Input: dimensioned drawing with shaded views. Units: mm. Origin: part minimum x, y, z. A direction names the side the tool comes from. Round coordinates to 2 decimals unless told otherwise and drop trailing zeros. Loops run counter-clockwise (first coordinate to the right, second up) from the corner with the lowest first, then second, coordinate; pieces in that order, holes last. Notation, with made-up numbers: (82, 62.25) -> (115, 62.25) arc R21 cw to (115, 99.25) -> close; hole circle Ø7 at (16.25, 40.25). An arc over 180 degrees is marked (long way). Answer as a JSON object with one key per item and string values.
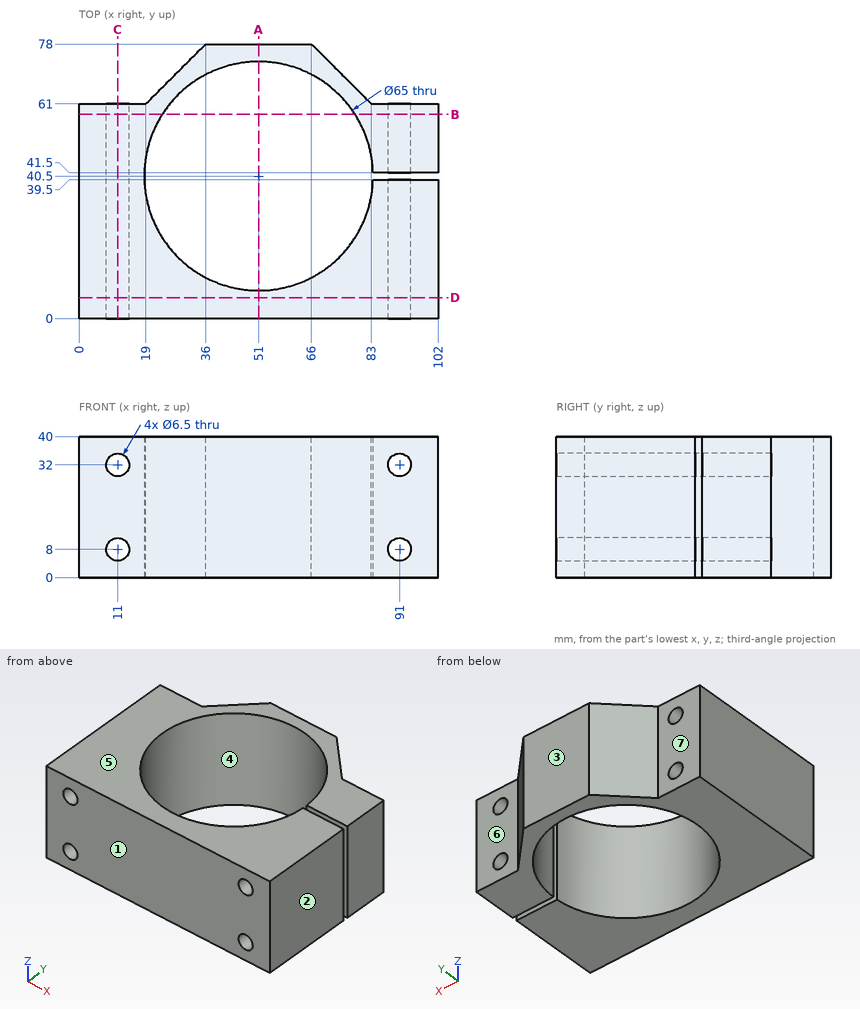
1) Reachability of the marked faces 5, 6 and 7 from +Z, -Z, +X, -X, +Y, -Y: full face, straight path, thin tool, end or side. Return the list, or none.
Output:
{"face 5": "+Z, +X, -X, +Y, -Y", "face 6": "+Z, -Z, +X, +Y", "face 7": "+Z, -Z, -X, +Y"}
2) Section B-B, the plane y = 58. Output: boundary loops of the cut face in (x, z).
Output:
{"outline": "(0, 0) -> (23.61, 0) -> (23.61, 40) -> (0, 40) -> close; (78.39, 0) -> (102, 0) -> (102, 40) -> (78.39, 40) -> close; hole circle Ø6.5 at (11, 8); hole circle Ø6.5 at (11, 32); hole circle Ø6.5 at (91, 8); hole circle Ø6.5 at (91, 32)"}
3) Draft query along Y for the marked faces 1, 2, 3 and 4. Return one class per face: +Y half, -Y half, draft (parallel to the pull), parting line (faces both ways), or undercut.
Output:
{"face 1": "-Y half", "face 2": "draft", "face 3": "+Y half", "face 4": "undercut"}
4) Ray query, probe 1 along X at (y, z) = (14, 32); probe 2 along Z at (x, y) = (8.5, 8); probe 3 along Y at (x, z) = (51, 15). Return the intervals inside material, ascending.
Output:
{"probe 1": "x = 0 to 7.75, 14.25 to 32.19, 69.81 to 87.75, 94.25 to 102", "probe 2": "z = 0 to 5.92, 10.08 to 29.92, 34.08 to 40", "probe 3": "y = 0 to 8, 73 to 78"}
5) Section C-C, the plane x = 11. Output: boundary loops of the cut face in (y, z), plus the area to 3 significant figures.
Output:
{"outline": "(0, 0) -> (61, 0) -> (61, 4.75) -> (0, 4.75) -> close; (0, 11.25) -> (61, 11.25) -> (61, 28.75) -> (0, 28.75) -> close; (0, 35.25) -> (61, 35.25) -> (61, 40) -> (0, 40) -> close", "area": "1,650 mm^2"}
6) Contact query for a flat-ended pin moving along its axis: P1, Ø15, axis at x = 7.5, z = 26.5, coming from the +Y side. Output: stop coordinate, or through.
Output:
{"P1": "stops at y = 61"}
7) Section A-A, the plane x = 51. Output: boundary loops of the cut face in (y, z), plus the area to 3 significant figures.
Output:
{"outline": "(0, 0) -> (8, 0) -> (8, 40) -> (0, 40) -> close; (73, 0) -> (78, 0) -> (78, 40) -> (73, 40) -> close", "area": "520 mm^2"}
8) Section D-D, the plane y = 6. Output: boundary loops of the cut face in (x, z), plus the area to 3 significant figures.
Output:
{"outline": "(0, 0) -> (102, 0) -> (102, 40) -> (0, 40) -> close; hole circle Ø6.5 at (11, 8); hole circle Ø6.5 at (11, 32); hole circle Ø6.5 at (91, 8); hole circle Ø6.5 at (91, 32)", "area": "3,950 mm^2"}
